For this review, use the dimensioned drawing (mm, ordinates from the lowest corner) and the shaded views. Give positions to 0.01 mm unless a question says otherwise; leave off trailing zeros. Write each loop counter-clockwise with the first axis right and the second up, starting at its lowest first coordinate (ties: lowest second). Pieces come first, ordered by that corner, then holes. Notation, with made-up numbers: (16, 81) -> (41, 81) arc R17 cw to (41, 113) -> close; hole circle Ø9 at (59.5, -17). An arc over 180 degrees is marked (long way). Return JSON: item names as keys, results as strings.
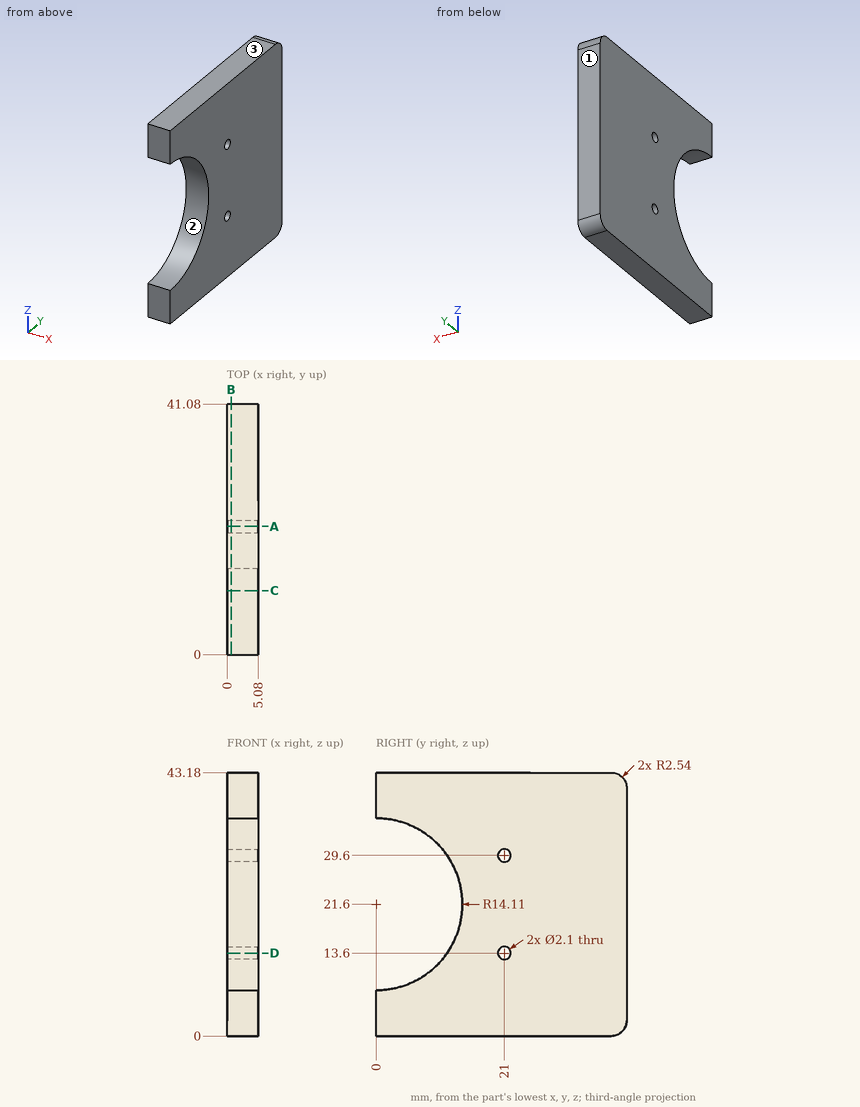
1. Add section D-D, the plane z = 13.6. State the section outline as (x, y) points, plus the area to 3 significant figures.
Results found:
{"outline": "(0, 11.62) -> (5.08, 11.62) -> (5.08, 19.95) -> (0, 19.95) -> close; (0, 22.05) -> (5.08, 22.05) -> (5.08, 41.08) -> (0, 41.08) -> close", "area": "139 mm²"}
2. Add section A-A, the plane y = 21. State the section outline as (x, z) points.
Results found:
{"outline": "(0, 0) -> (5.08, 0) -> (5.08, 12.55) -> (0, 12.55) -> close; (0, 14.65) -> (5.08, 14.65) -> (5.08, 28.55) -> (0, 28.55) -> close; (0, 30.65) -> (5.08, 30.65) -> (5.08, 43.18) -> (0, 43.18) -> close"}
3. Add section C-C, the plane y = 10.5. State the section outline as (x, z) points (1 decimal).
Results found:
{"outline": "(0, 0) -> (5.1, 0) -> (5.1, 12.2) -> (0, 12.2) -> close; (0, 31) -> (5.1, 31) -> (5.1, 43.2) -> (0, 43.2) -> close"}
4. The part is to be moulded in two halves that separate along Z. For the marked faces 1, 2 and 3, say which applies: +Z half, -Z half, draft (parallel to the pull), parting line (faces both ways), or undercut.
Results found:
{"face 1": "draft", "face 2": "undercut", "face 3": "+Z half"}
5. To check wall thickness, follow probe 1 along Z at (x, y) = (4.25, 21.5); probe 2 along Y at (x, z) = (3.9, 13.6); probe 3 along Z at (x, y) = (2.5, 8.5). State the ranges of each line that lie inside material, in increasing order.
Results found:
{"probe 1": "z = 0 to 12.68, 14.52 to 28.68, 30.52 to 43.18", "probe 2": "y = 11.62 to 19.95, 22.05 to 41.08", "probe 3": "z = 0 to 10.34, 32.86 to 43.18"}
6. Add section B-B, the plane x = 0.65. State the section outline as (y, z) points, plus the area to 3 significant figures.
Results found:
{"outline": "(0, 0) -> (38.54, 0) arc R2.54 ccw to (41.08, 2.54) -> (41.08, 40.64) arc R2.54 ccw to (38.54, 43.18) -> (0, 43.18) -> (0, 35.71) arc R14.11 cw to (0, 7.49) -> close; hole circle Ø2.1 at (21, 13.6); hole circle Ø2.1 at (21, 29.6)", "area": "1,450 mm²"}
